Part model, mm, in its own coordinate system. A direction names the side the tool comes from. Coordinates: 2 decimals unless noted, no trailing zeros. Loops run counter-clockwise (first coordinate to the right, second up) from the corner with the lowest first, then second, coordinate; pieces in that order, holes last. Notation, with made-up numbers: (21.25, -19) - (60.25, -19) arc R18 ccw to (60.25, -11) - close; hole circle Ø8 at (39, 13). An arc over 180 degrees is marked (long way). Use a Markdown table: item, result. Add a question column.
1. Band-saw the part on C-C, the plane x = -3.25. Give the cut face in (y, z) (3 decimals), plus the area to 3 significant figures.
2. Band-saw the part on A-A, the plane y = 0. Give the cut face in (x, z) (3 decimals), plus the area to 3 significant figures.
3. Band-saw the part on B-B, the plane z = -0.5. Give the cut face in (x, y), plus the area to 3 significant figures.
4. Drop flat-ended pins along their axis: pin 1 (3 mm diameter, centred on x = -3.5, z = -13, fed in from -Y); pin 2 (1 mm diameter, centred on y = -2, z = -21.5, fed in from -X); pin 3 (2 mm diameter, centred on y = 3, z = -20.5, fed in from -X). Give the stop position or say it passes through.
5. 3-axis set-ups, long thin cutter, end or side, ignore diameter. For faces 1 (the cylindrical face through (3.785, 1.192, -1.565)), 2 (the flat face through (-6.28, 0, 3)): which of +Z, -Z, +X, -X, +Y, -Y reach the whole face in a straight line?
6. Wall check: probe 1 along Y at (x, z) = (1.5, -7.5); probe 2 along Z at (x, y) = (-3.25, 2.5); probe 3 along X at (y, z) = (1.75, -21.5). Give the ranges that are in metal, low to high. Write a range as [from, to].
7. Band-saw the part on D-D, the plane z = -9. Give the cut face in (x, y).
from build123d import *

# Parameters (mm, degrees)
HEAD_DEPTH     = 5.1562
SHANK_SKETCH_R = 3.96875
SHANK_DEPTH    = 25.4
THREAD_END_W   = 22.225
THREAD_END_H   = 0.05


with BuildPart() as part:
    # Head Sketch → Head (new body)
    with BuildSketch(Plane.XY):
        Polygon((0, 7.251692586), (6.28015, 3.625846293), (6.28015, -3.625846293), (0, -7.251692586), (-6.28015, -3.625846293), (-6.28015, 3.625846293), align=None)
    extrude(amount=HEAD_DEPTH)

    # Shank Sketch → Shank (add)
    with BuildSketch(Plane.XY):
        Circle(SHANK_SKETCH_R)
    extrude(amount=-SHANK_DEPTH)

    # Thread End → Thread Cut (revolve, cut)
    with BuildSketch(Plane(origin=(0, 0, 0), x_dir=(0, 0, -1), z_dir=(1, 0, 0))):
        with Locations((14.2875, 3.94375)):
            Rectangle(THREAD_END_W, THREAD_END_H)
    revolve(axis=Axis((0, 0, -21.551935625), (0, 0, -1)), mode=Mode.SUBTRACT)


solid = part.part
Geometry check:
| question | item | result |
|---|---|---|
| 1 | outline | (-5.375, 0) - (-2.278, 0) - (-2.278, -3.175) - (-2.19, -3.175) - (-2.19, -25.4) - (2.19, -25.4) - (2.19, -3.175) - (2.278, -3.175) - (2.278, 0) - (5.375, 0) - (5.375, 5.156) - (-5.375, 5.156) - close |
| 1 | area | 167 mm^2 |
| 2 | outline | (-6.28, 0) - (-3.969, 0) - (-3.969, -3.175) - (-3.919, -3.175) - (-3.919, -25.4) - (3.919, -25.4) - (3.919, -3.175) - (3.969, -3.175) - (3.969, 0) - (6.28, 0) - (6.28, 5.156) - (-6.28, 5.156) - close |
| 2 | area | 264 mm^2 |
| 3 | outline | circle Ø7.94 at (0, 0) |
| 3 | area | 49.5 mm^2 |
| 4 | pin 1 | stops at y = -3.37 |
| 4 | pin 2 | stops at x = -3.62 |
| 4 | pin 3 | stops at x = -3.37 |
| 5 | face 1 | -Z |
| 5 | face 2 | +Z, -Z, -X, +Y, -Y |
| 6 | probe 1 | y = [-3.62, 3.62] |
| 6 | probe 2 | z = [0, 5.16] |
| 6 | probe 3 | x = [-3.51, 3.51] |
| 7 | outline | circle Ø7.84 at (0, 0) |
